Source: three-view drawing plus pictorial views. Frame: mm from the lowest corner of the part. Coordinates: 2 decimals unless noted, no trailing zeros. Loops run counter-clockwise (first coordinate to the right, second up) from the corner with the lowest first, then second, coordinate; pieces in that order, holes last.
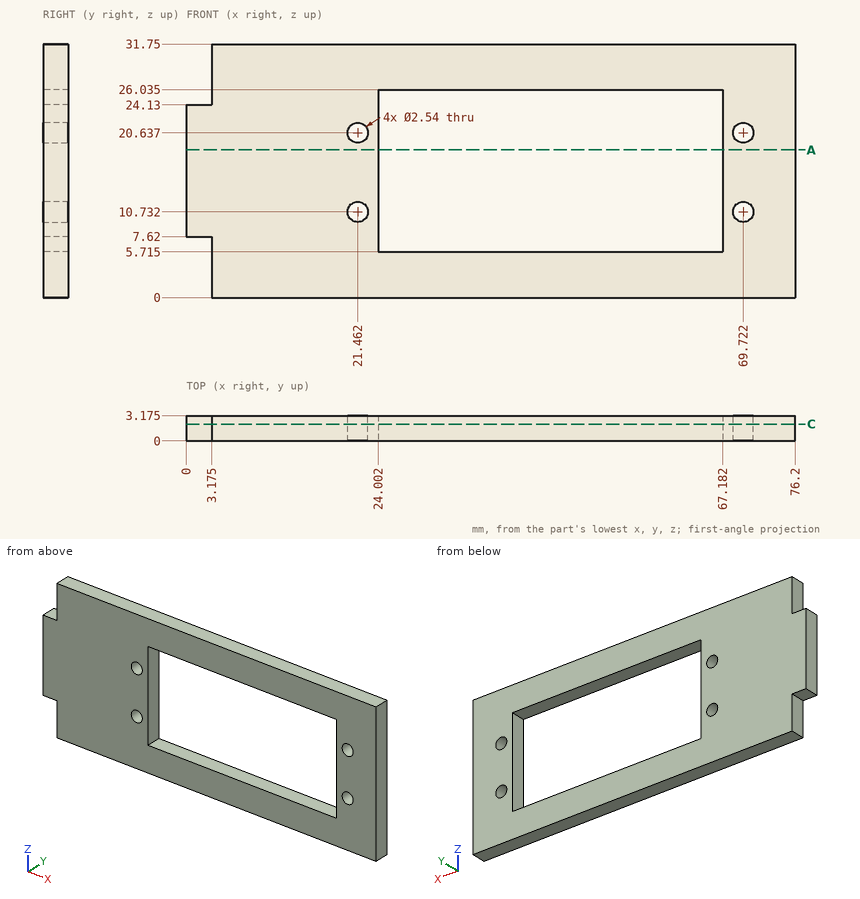
Q1. Contact query for flat-ended pins moving along their axis: pin 1 Ø1.6 at (y, z) = (1.5, 28) entering from -X (1 decimal); pin 2 Ø1 at (y, z) = (1, 12.5) entering from -X; pin 3 Ø2 at (x, z) = (21.46, 20.64) entering from +Y. Output: stop coordinate, or through.
Q2. Line query: line 1 along Z through (x, y) = (21.5, 1.3); line 2 along X through (y, z) = (1.3, 17); line 3 along X through (y, z) = (1.6, 4) (1 decimal). Output: solid intervals per line, ascending.
Q3. Section A-A, the plane z = 18.5. Return the cut outline in (x, y) (1 decimal).
Q4. Section C-C, the plane y = 2.1. Count the separate pieces of the cut face and the enclosed holes in it, plus the area to 3 significant figures.
Derived:
1. pin 1: stops at x = 3.2
1. pin 2: stops at x = 0
1. pin 3: passes through
2. line 1: z = 0 to 9.46, 12 to 19.37, 21.91 to 31.75
2. line 2: x = 0 to 24, 67.18 to 76.2
2. line 3: x = 3.2 to 76.2
3. outline: (0, 0) - (24, 0) - (24, 3.2) - (0, 3.2) - close; (67.2, 0) - (76.2, 0) - (76.2, 3.2) - (67.2, 3.2) - close
4. separate pieces: 1
4. enclosed holes: 5
4. area: 1,470 mm2
